The figure shows three views and two pictorial views of one solid part (mm, origin at its lowest corner). Answer the questions. A direction names the side the tool comes from. Give positions to 0.01 mm unless a question says otherwise; leave off trailing zeros. Loops run counter-clockwise (first coordinate to the right, second up) from the corner with the lowest first, then second, coordinate; pieces in that order, holes last. Notation, with made-up numbers: (38.25, 51) - (69.25, 51) arc R29 ccw to (69.25, 83) - close; hole circle Ø4 at (43, 75). An arc over 180 degrees is marked (long way). Use CSV: the item, a comma, the result in double quotes.
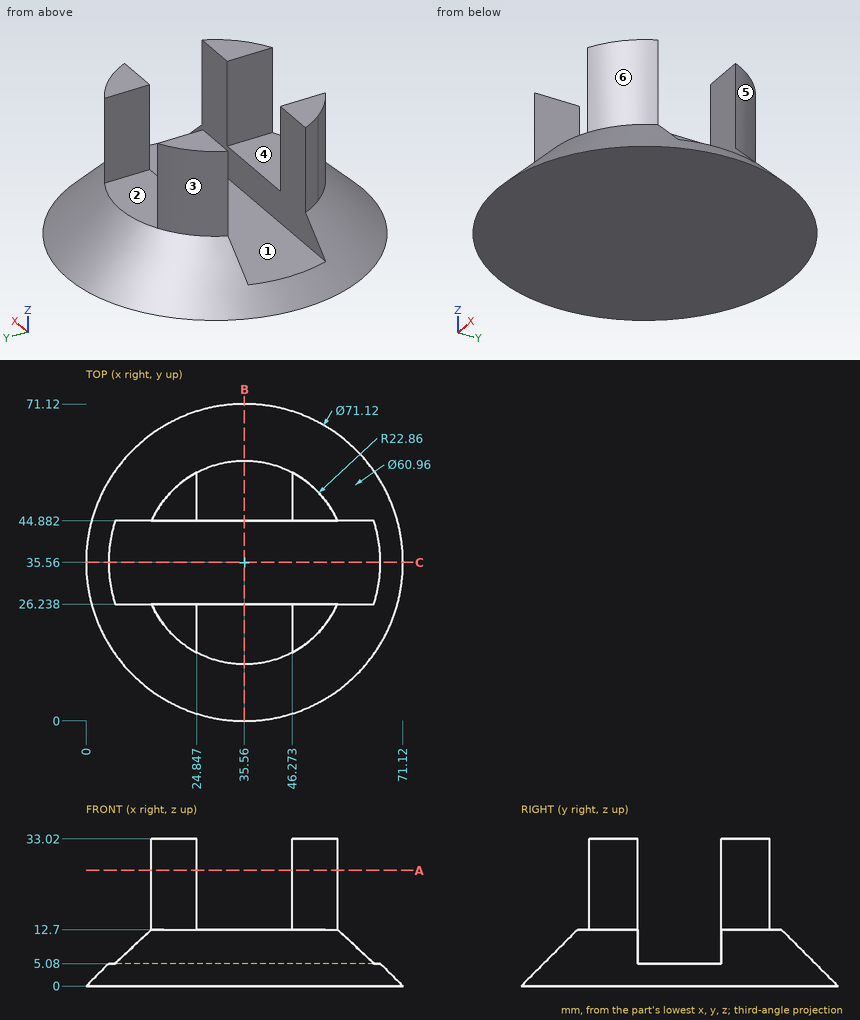
Item 1: A cutting plane is placed at A-A on z = 26. Determine the outline of the cut face in (x, y).
Determined:
outline,"(14.69, 26.24) arc R22.86 ccw to (24.85, 15.37) - (24.85, 26.24) - close; (14.69, 44.88) - (24.85, 44.88) - (24.85, 55.75) arc R22.86 ccw to start; (46.27, 15.37) arc R22.86 ccw to (56.43, 26.24) - (46.27, 26.24) - close; (46.27, 44.88) - (56.43, 44.88) arc R22.86 ccw to (46.27, 55.75) - close"
Item 2: For the marked faces 4, 5 and 6, determine the directions among +Z, -Z, +X, -X, +Y, -Y from which every point of the face is accessible in a straight line to the end or side of a thin tool.
Determined:
face 4,"+Z, +Y, -Y"
face 5,"+Z, +X, +Y"
face 6,"+Z, +X, -Y"
Item 3: Find the intervals of material crossed by line 1 (X direction, y = 52, z = 25.5) (1 decimal); line 2 (Z direction, x = 42.5, y = 56); line 3 (Y direction, x = 52, z = 30.5) (1 decimal), in increasing order.
Determined:
line 1,"x = 19.7 to 24.8, 46.3 to 51.4"
line 2,"z = 0 to 12.7"
line 3,"y = 19.7 to 26.2, 44.9 to 51.4"
Item 4: The mould has two halves that part along Y. Classify the marked faces 1, 2 and 3: pulls with the +Y half, pulls with the -Y half, needs draft (parallel to the pull), parting line crosses it, or undercut.
Determined:
face 1,"undercut"
face 2,"needs draft"
face 3,"pulls with the +Y half"
Item 5: Given P1, Ø5.5, axis at y = 50.5, z = 28, coming from the +X side; P2, Ø5.5, axis at y = 21, z = 23, coming from the -X side; P3, Ø12, axis at y = 51.5, z = 23.5, coming from the -X side; P4, Ø12, axis at x = 11.5, y = 13.5, coming from the -Z side, each flat-ended and moving along its own axis, determine where each tip first touches the part or whether it passes through.
Determined:
P1,"stops at x = 54.9"
P2,"stops at x = 15.99"
P3,"stops at x = 14.97"
P4,"stops at z = 0"
Item 6: A cutting plane is placed at B-B on x = 35.56. Determine the outline of the cut face in (y, z), and give its area (3 significant figures).
Determined:
outline,"(0, 0) - (71.12, 0) - (58.42, 12.7) - (44.88, 12.7) - (44.88, 5.08) - (26.24, 5.08) - (26.24, 12.7) - (12.7, 12.7) - close"
area,"600 mm²"
Item 7: A cutting plane is placed at C-C on y = 35.56. Determine the outline of the cut face in (x, z).
Determined:
outline,"(0, 0) - (71.12, 0) - (66.04, 5.08) - (5.08, 5.08) - close"
